from build123d import *

# Parameters (mm, degrees)
SKETCH1_W           = 50.8
SKETCH1_H           = 152.4
BOSS_EXTRUDE1_DEPTH = 5.9436
SKETCH2_R           = 1.1303
SKETCH2_W           = 20.7
SKETCH2_H           = 41.3
CUT_EXTRUDE1_DEPTH  = 6.9436


with BuildPart() as part:
    # Sketch1 → Boss-Extrude1 (new body)
    with BuildSketch(Plane.XY):
        with Locations((25.4, 76.2)):
            Rectangle(SKETCH1_W, SKETCH1_H)
    extrude(amount=BOSS_EXTRUDE1_DEPTH)

    # Sketch2 → Cut-Extrude1 (cut, through all)
    with BuildSketch(Plane.XY.offset(5.9436)):
        with Locations((20.492131346, 116.1)):
            Circle(SKETCH2_R)
        with Locations((30.492131346, 116.1)):
            Circle(SKETCH2_R)
        with Locations((20.492131346, 65.8)):
            Circle(SKETCH2_R)
        with Locations((30.492131346, 65.8)):
            Circle(SKETCH2_R)
        with Locations((25.492131346, 90.95)):
            Rectangle(SKETCH2_W, SKETCH2_H)
    extrude(amount=-CUT_EXTRUDE1_DEPTH, mode=Mode.SUBTRACT)


solid = part.part
The model under review builds one solid part; all positions refer to its coordinate system, in mm. A direction names the side the tool comes from. Round coordinates to 2 decimals unless told otherwise and drop trailing zeros. Order: outer loops, then holes, each group sorted by start corner. A loop starts at its lowest first (then second) coordinate and runs counter-clockwise, first axis right, second up. Notation, with made-up numbers: (-5.5, 41) -> (15.5, 41) arc R9 cw to (15.5, 50) -> close; hole circle Ø3 at (-6, -27.75). An arc over 180 degrees is marked (long way). Use CSV: the item, a comma, the result in double quotes. Start each with the question number.
(1) Tool access review of faces 1 (the face through (0, 75, 3)), 2 (the face through (15.142, 91, 3)): name each direction out of +Z, -Z, +X, -X, +Y, -Y from which nothing blocks a thin tool from reaching the whole face with its end or side.
(2) Consider section C-C on z = 1.5. Write out the cut boundary in (x, y), and give its area (3 significant figures).
(3) Consider section B-B on x = 16.5. Write out the cut boundary in (y, z).
(4) Wall thickness on probe 1 along X at (y, z) = (65.8, 2.25); probe 2 along Y at (x, z) = (31, 0.5); probe 3 along Y at (x, z) = (19, 1.75): over which ranges is each line inside the solid? List them lowest first. Write a range as from..to.
(5) Mouldability with a two-part tool opening along Y and no side actions: class faces 3 (the face through (50.8, 75, 3)), 4 (the face through (25, 152.4, 3)), 5 (the face through (35.842, 91, 3)), 6 (the face through (25, 70.3, 3)) as pulls with the +Y half, pulls with the -Y half, needs draft (parallel to the pull), parting line crosses it, or undercut.
(6) Consider section A-A on y = 90.5. Write out the cut boundary in (x, z).
(7) Insertion check: pin 1 (3 mm diameter, centred on x = 28.5, z = 4.5, fed in from -Y). The pin has a flat end and moves straight along its axis. Give the tip position at first contact, or say it passes through.
Responses:
1,face 1,"+Z, -Z, -X, +Y, -Y"
1,face 2,"+Z, -Z"
2,outline,"(0, 0) -> (50.8, 0) -> (50.8, 152.4) -> (0, 152.4) -> close; hole (15.14, 70.3) -> (35.84, 70.3) -> (35.84, 111.6) -> (15.14, 111.6) -> close; hole circle Ø2.26 at (20.49, 65.8); hole circle Ø2.26 at (20.49, 116.1); hole circle Ø2.26 at (30.49, 65.8); hole circle Ø2.26 at (30.49, 116.1)"
2,area,"6,870 mm²"
3,outline,"(0, 0) -> (70.3, 0) -> (70.3, 5.94) -> (0, 5.94) -> close; (111.6, 0) -> (152.4, 0) -> (152.4, 5.94) -> (111.6, 5.94) -> close"
4,probe 1,"0..19.36, 21.62..29.36, 31.62..50.8"
4,probe 2,"0..64.79, 66.81..70.3, 111.6..115.09, 117.11..152.4"
4,probe 3,"0..70.3, 111.6..152.4"
5,face 3,"needs draft"
5,face 4,"pulls with the +Y half"
5,face 5,"undercut"
5,face 6,"undercut"
6,outline,"(0, 0) -> (15.14, 0) -> (15.14, 5.94) -> (0, 5.94) -> close; (35.84, 0) -> (50.8, 0) -> (50.8, 5.94) -> (35.84, 5.94) -> close"
7,pin 1,"y = 0"
